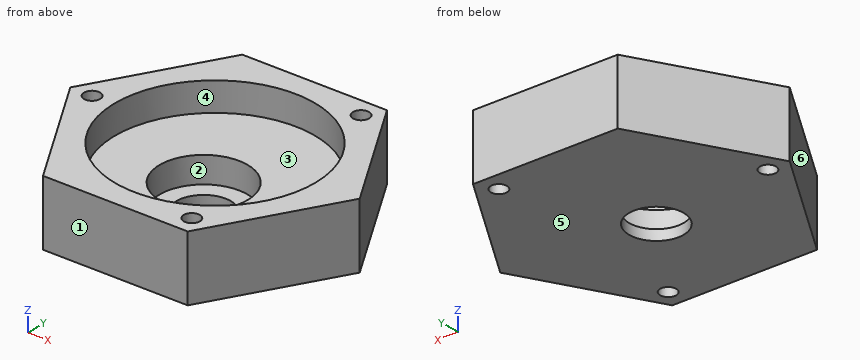
Autodesk Inventor part; units mm, degrees
ref_plane "Work Plane1" through (0, 0, 12.5) normal (0, 0, 1) x (1, 0, 0)
ref_plane "YZ Plane" through (0, 0, 0) normal (1, 0, 0) x (0, 1, 0)
ref_plane "XZ Plane" through (0, 0, 0) normal (0, 1, 0) x (-1, 0, 0)
sketch "Sketch1" plane through (0, 0, 0) normal (0, 0, 1) x (1, 0, 0)
  circle A0 centre (0, 0) radius 19.2
  line L0 (-13.6832, 23.7) -> (13.6832, 23.7)
  line L1 (13.6832, 23.7) -> (27.3664, 0)
  line L2 (27.3664, 0) -> (13.6832, -23.7)
  line L3 (13.6832, -23.7) -> (-13.6832, -23.7)
  line L4 (-13.6832, -23.7) -> (-27.3664, 0)
  line L5 (-27.3664, 0) -> (-13.6832, 23.7)
  circle A1 centre (11.6207, 20.1277) radius 1.55
  line L6 (0, 23.7) -> (0, 19.2) construction
  circle A2 centre (0, -2.7) radius 5.25
  circle A3 centre (0, -2.7) radius 8.45
  line L7 (11.6207, 20.1277) -> (9.6, 16.6277) construction
  circle A4 centre (-23.2415, 0) radius 1.55
  circle A5 centre (11.6207, -20.1277) radius 1.55
  point P0 (0, 21.45)
  point P1 (0, -19.2)
  dimension "d1" = 3.1
  dimension "d2" = 4.5
  dimension "d23" = 10.5
  dimension "d24" = 16.9
  dimension "d46" = 3.5
  dimension "d47" = -30
  dimension "d50" = 360
  dimension "d53" = 16.5
  dimension "d54" = 2.7
extrude "Extrusion1" add sketch "Sketch1" along normal blind 2 contours A3
extrude "Extrusion2" add sketch "Sketch1" along normal blind 7 contours A0
extrude "Extrusion3" add sketch "Sketch1" along normal blind 12.5 contours L0 L1 L2 L3 L4 L5
sketch "Sketch2" plane through (0, 0, 12.5) normal (0, 0, 1) x (1, 0, 0)
  circle A0 centre (0, 0) radius 19.2
  line L0 (0, -19.2) -> (0, -23.7) construction
  line L1 (-13.6832, -23.7) -> (13.6832, -23.7)
  line L2 (-11.0127, -15.7277) -> (-14.9991, -21.4209) construction
  line L3 (-18.2603, -5.9331) -> (-23.0436, -7.4873) construction
  line L4 (9.6, 16.6277) -> (13.6832, 23.7)
  line L5 (13.5765, -13.5765) -> (17.3496, -17.3496)
  line L6 (13.6832, -23.7) -> (27.3664, 0)
  line L7 (27.3664, 0) -> (13.6832, 23.7)
  line L8 (-27.3664, 0) -> (-13.6832, -23.7)
  circle A1 centre (0, -2.7) radius 5.25
  line L9 (-11.0127, -15.7277) -> (-13.1923, -18.8405)
  arc A2 (-18.2603, -5.9331) -> (-13.1923, -18.8405) centre (91.7215, 29.8021) ccw
  dimension "d15" = 35
  dimension "d16" = 72
  dimension "d18" = 150
  dimension "d19" = 45
  dimension "d45" = 3.8
ref_plane "Work Plane1" through (0, 0, 12.5) normal (0, 0, 1) x (1, 0, 0)
sketch "Sketch3" plane through (0, 0, 12.5) normal (0, 0, 1) x (1, 0, 0)
  line L0 (-12.6187, -18.0213) -> (7.041, -31.7872)
  line L1 (-11.1058, -22.8345) -> (5.2772, -34.3061)
  line L2 (-11.1058, -22.8345) -> (-13.1923, -18.8405)
  line L3 (5.2772, -34.3061) -> (7.041, -31.7872)
  line L4 (-12.6187, -18.0213) -> (-13.1923, -18.8405)
  line L5 (-11.0127, -15.7277) -> (-13.1923, -18.8405)
  point P0 (0, 0)
  dimension "d36" = 6.15
  dimension "d41" = 20
  dimension "d43" = 2
  dimension "d55" = 4
properties part number "Case V2"
Input: part model. Units: mm. Frame: model coordinates. Face numbers are marked on the shaded views. A direction names the side the tool comes from. Coordinates: 2 decimals unless noted, no trailing zeros. Loops run counter-clockwise (first coordinate to the right, second up) from the corner with the lowest first, then second, coordinate; pieces in that order, holes last.
(1) Pull-direction query (Y, two-part tool) for the marked faces 3, 4, 5 and 6; classes: released by +Y, released by -Y, zero draft, split by the parting line, or undercut.
(2) Section A-A on x = 0. Return the cut outline in (y, z).
(3) Section B-B on y = -2.7. Return the cut outline in (x, z), then the cut area to 3 significant figures.
(4) First-contact query: pin 1 Ø22 at (x, y) = (0, -2.7) entering from +Z; pin 2 Ø5 at (x, y) = (-3.5, -1.5) entering from +Z; pin 3 Ø4 at (y, z) = (-8.5, 3) entering from +X; pin 4 Ø1.9 at (x, y) = (11.62, 20.13) entering from +Z. Flat tips, straight axial feed; report the tip coordinate or a pass-through.
(5) Section D-D on x = 16.5. Return the cut outline in (y, z).
(6) Section C-C on z = 11.5. Return the cut outline in (x, y), then the cut area to 3 significant figures.
(7) Set-up query: the marked faces 1 and 2. Return all of +Z, -Z, +X, -X, +Y, -Y with unobstructed straight access to the full face (end or side cutting, diameter ignored); none if empty.
(8) Material intervals for probe 1 along Y at (x, z) = (0, 1.35); probe 2 along Y at (x, z) = (-2, 5.5); probe 3 along Z at (x, y) = (-5, -10), sorted ascending.
Data:
1. face 3: undercut
1. face 4: undercut
1. face 5: zero draft
1. face 6: released by -Y
2. outline: (-23.7, 0) - (-7.95, 0) - (-7.95, 2) - (-11.15, 2) - (-11.15, 7) - (-19.2, 7) - (-19.2, 12.5) - (-23.7, 12.5) - close; (2.55, 0) - (23.7, 0) - (23.7, 12.5) - (19.2, 12.5) - (19.2, 7) - (5.75, 7) - (5.75, 2) - (2.55, 2) - close
3. outline: (-25.81, 0) - (-5.25, 0) - (-5.25, 2) - (-8.45, 2) - (-8.45, 7) - (-19.01, 7) - (-19.01, 12.5) - (-25.81, 12.5) - close; (5.25, 0) - (25.81, 0) - (25.81, 12.5) - (19.01, 12.5) - (19.01, 7) - (8.45, 7) - (8.45, 2) - (5.25, 2) - close
3. area: 331 mm2
4. pin 1: stops at z = 7
4. pin 2: stops at z = 2
4. pin 3: stops at x = 23.61
4. pin 4: passes through
5. outline: (-18.82, 0) - (18.82, 0) - (18.82, 12.5) - (9.82, 12.5) - (9.82, 7) - (-9.82, 7) - (-9.82, 12.5) - (-18.82, 12.5) - close
6. outline: (-27.37, 0) - (-13.68, -23.7) - (13.68, -23.7) - (27.37, 0) - (13.68, 23.7) - (-13.68, 23.7) - close; hole circle Ø3.1 at (-23.24, 0); hole circle Ø38.4 at (0, 0); hole circle Ø3.1 at (11.62, -20.13); hole circle Ø3.1 at (11.62, 20.13)
6. area: 765 mm2
7. face 1: +Z, -Z, +X, -X, -Y
7. face 2: +Z
8. probe 1: y = -23.7 to -7.95, 2.55 to 23.7
8. probe 2: y = -23.7 to -10.91, 5.51 to 23.7
8. probe 3: z = 0 to 7
